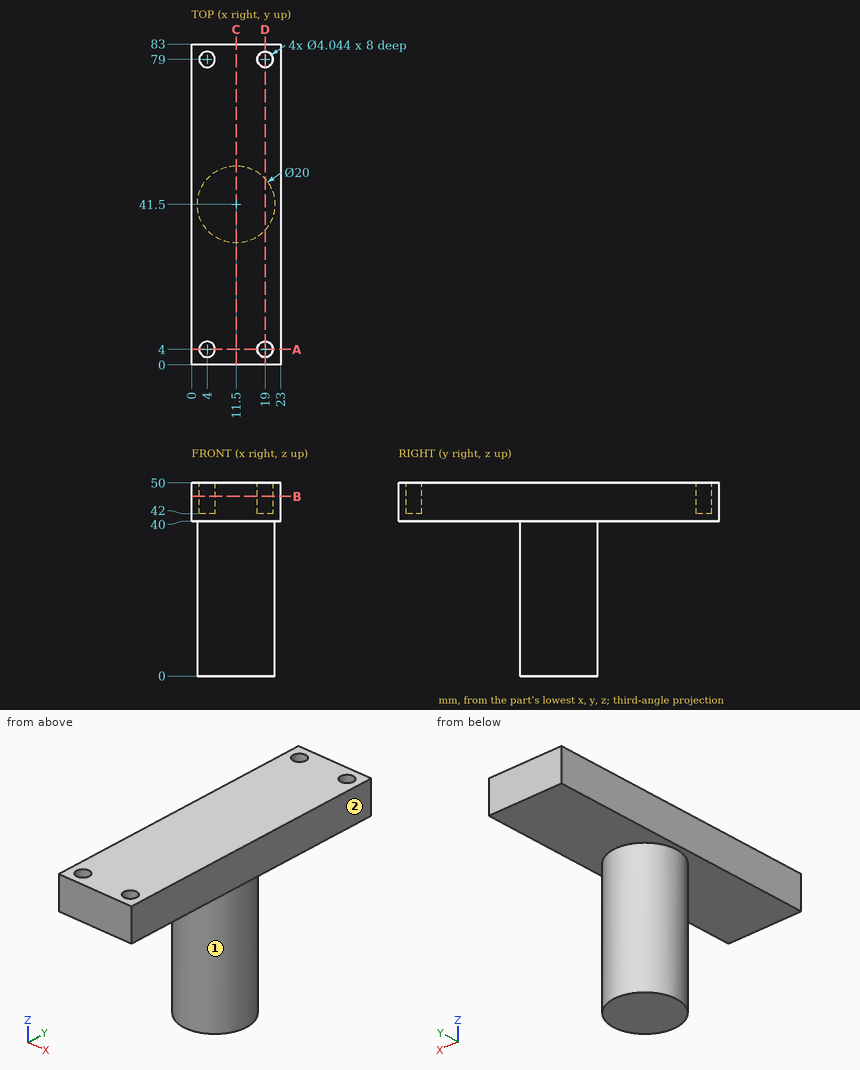
Design review of the part shown in the three views and the two pictorial views. Dimensions are in mm from the part's minimum x, y and z. A direction names the side the tool comes from. Round coordinates to 2 decimals unless told otherwise and drop trailing zeros. Write each loop counter-clockwise with the first axis right and the second up, starting at its lowest first coordinate (ties: lowest second). Pieces come first, ordered by that corner, then holes. Notation, with made-up numbers: (81.25, 53) -> (93.25, 53) arc R31 ccw to (93.25, 84) -> close; hole circle Ø6 at (-31, 85). An arc over 180 degrees is marked (long way). One line per question, with ' | ' between items. Start each with the question number.
1) Machinability: for the marked faces 1 and 2, which of the approach directions +Z, -Z, +X, -X, +Y, -Y give a long, thin tool a straight path to every point of the face, cutting with its end or side? Answer none if there is none.
2) Add section B-B (z = 46.5). Write out the cut boundary in (x, y), and give its area (3 significant figures).
3) Add section C-C (x = 11.5). Write out the cut boundary in (y, z), and give its area (3 significant figures).
4) For pin 1 Ø5 at (x, z) = (7, 25.5) entering from -Y; pin 2 Ø12 at (x, y) = (6.5, 58.5) entering from -Z; pin 3 Ø1.2 at (x, y) = (19, 79) entering from +Z, all flat-tipped, find the tip position at first contact; note any pin that passes through.
5) Add section D-D (x = 19). Write out the cut boundary in (y, z).
6) Wall thickness on line 1 along Y through (x, z) = (4, 45); line 2 along Y through (x, z) = (3, 47.5); line 3 along Z through (x, y) = (16, 70): over which ranges is each line inside the solid? List them lowest first.
7) Add section A-A (y = 4). Write out the cut boundary in (x, z), and give its area (3 significant figures).
Reported:
1) face 1: -Z | face 2: +Z, -Z, +X, +Y, -Y
2) outline: (0, 0) -> (23, 0) -> (23, 83) -> (0, 83) -> close; hole circle Ø4.04 at (4, 4); hole circle Ø4.04 at (4, 79); hole circle Ø4.04 at (19, 4); hole circle Ø4.04 at (19, 79) | area: 1,860 mm²
3) outline: (0, 40) -> (31.5, 40) -> (31.5, 0) -> (51.5, 0) -> (51.5, 40) -> (83, 40) -> (83, 50) -> (0, 50) -> close | area: 1,630 mm²
4) pin 1: stops at y = 31.7 | pin 2: stops at z = 40 | pin 3: stops at z = 42
5) outline: (0, 40) -> (34.89, 40) -> (34.89, 0) -> (48.11, 0) -> (48.11, 40) -> (83, 40) -> (83, 50) -> (81.02, 50) -> (81.02, 42) -> (76.98, 42) -> (76.98, 50) -> (6.02, 50) -> (6.02, 42) -> (1.98, 42) -> (1.98, 50) -> (0, 50) -> close
6) line 1: y = 0 to 1.98, 6.02 to 76.98, 81.02 to 83 | line 2: y = 0 to 2.24, 5.76 to 77.24, 80.76 to 83 | line 3: z = 40 to 50
7) outline: (0, 40) -> (23, 40) -> (23, 50) -> (21.02, 50) -> (21.02, 42) -> (16.98, 42) -> (16.98, 50) -> (6.02, 50) -> (6.02, 42) -> (1.98, 42) -> (1.98, 50) -> (0, 50) -> close | area: 165 mm²
